Here's how the part is built. I have some questions about the finished solid (model axes, mm). Face numbers are marked on the shaded views. Coordinates: 2 decimals unless noted, no trailing zeros. Write each loop counter-clockwise with the first axis right and the second up, starting at its lowest first coordinate (ties: lowest second). Pieces come first, ordered by that corner, then holes. Notation, with made-up numbers: (7, 66) -> (66, 66) arc R12 ccw to (66, 86) -> close; hole circle Ø7 at (-7, 36.5). An arc over 180 degrees is marked (long way). Put each result on its own line as item: value. Start each with the question number.
Item 1: I want a section at D-D, the plane x = 113. List the corners of the cut face in (y, z) for me, then the cut area to 3 significant figures.
Item 2: If we mould it in two halves opening along Y, with no side actions, what happens to the marked faces 1 and 2? For each: released by +Y, released by -Y, zero draft, split by the parting line, or undercut.
Item 3: I want a section at C-C, the plane y = 32. List the corners of the cut face in (x, z) for me.
Item 4: For pin 1 (2 mm diameter, centred on x = 151.5, y = 38.5, fed in from -Z); pin 2 (10 mm diameter, centred on x = 61, y = 61.5, fed in from -Z), each with a flat end and sliding along its axis, tell me the tip position at first contact or that it passes through.
Item 5: I want a section at A-A, the plane x = 18. List the corners of the cut face in (y, z) for me, then the cut area to 3 significant figures.
Item 6: I want a section at B-B, the plane z = 3. State how many separate pieces and enclosed holes the cut face has, then the cut area to 3 significant figures.
Item 7: I need wall thicknesses on line 1 (Y direction, x = 27.75, z = 2.25); line 2 (X direction, y = 63, z = 4.75); line 3 (X direction, y = 16, z = 7.25). Which ranges of each line are inside material? Lowest first, please. Write a range as [from, to].
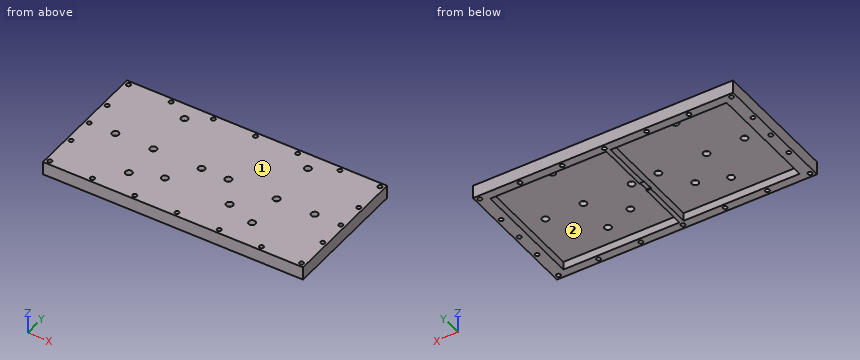
from build123d import *

# Parameters (mm, degrees)
F0_W      = 154
F0_H      = 77
F1_DEPTH  = 7.873
F2_W      = 140
F2_H      = 67
F3_DEPTH  = 4.873
F4_R      = 1.25
F5_DEPTH  = 7.873
F6_R      = 1.25
F7_DEPTH  = 7.873
F8_R      = 1.25
F9_DEPTH  = 7.873
F10_R     = 1.25
F11_DEPTH = 7.873
F12_R     = 1.25
F13_DEPTH = 7.873
F14_R     = 1.25
F15_DEPTH = 7.873
F16_R     = 1.25
F17_DEPTH = 7.873
F18_R     = 1.25
F19_DEPTH = 7.873
F20_R     = 1.25
F21_DEPTH = 7.873
F22_R     = 1.25
F23_DEPTH = 7.873
F24_R     = 1.25
F25_DEPTH = 7.873
F26_R     = 1.25
F27_DEPTH = 7.873
F28_R     = 1.25
F29_DEPTH = 7.873
F30_R     = 1.25
F31_DEPTH = 7.873
F32_R     = 1.25
F33_DEPTH = 7.873
F34_R     = 1.25
F35_DEPTH = 7.873
F36_R     = 1.25
F37_DEPTH = 7.873
F38_R     = 1.25
F39_DEPTH = 7.873
F40_R     = 1.25
F41_DEPTH = 7.873
F42_R     = 1.25
F43_DEPTH = 7.873
F44_R     = 2
F45_DEPTH = 3
F46_R     = 2
F47_DEPTH = 3
F48_R     = 2
F49_DEPTH = 3
F50_R     = 2
F51_DEPTH = 3
F52_R     = 2
F53_DEPTH = 3
F54_R     = 2
F55_DEPTH = 3
F56_R     = 2
F57_DEPTH = 3
F58_R     = 2
F59_DEPTH = 3
F61_R     = 2
F62_DEPTH = 3
F64_R     = 2
F65_DEPTH = 3
F66_R     = 2
F67_DEPTH = 3
F63_R     = 2
F68_DEPTH = 3
F69_W     = 2.5
F69_H     = 67
F70_DEPTH = 4.873
F60_W     = 2.5
F60_H     = 6.7
F71_DEPTH = 0.723


with BuildPart() as f1:
    # F0 (on Top) → F1 (new body)
    with BuildSketch(Plane.XY):
        with Locations((77, 38.5)):
            Rectangle(F0_W, F0_H)
    extrude(amount=F1_DEPTH)

    # F2 (on Top) → F3 (cut)
    with BuildSketch(Plane.XY):
        with Locations((77, 38.5)):
            Rectangle(F2_W, F2_H)
    extrude(amount=F3_DEPTH, mode=Mode.SUBTRACT)

    # F4 (on face) → F5 (cut)
    with BuildSketch(Plane.XY.offset(7.873)):
        with Locations((2.5, 2.5)):
            Circle(F4_R)
    extrude(amount=-F5_DEPTH, mode=Mode.SUBTRACT)

    # F6 (on face) → F7 (cut)
    with BuildSketch(Plane.XY.offset(7.873)):
        with Locations((27.75, 2.5)):
            Circle(F6_R)
    extrude(amount=-F7_DEPTH, mode=Mode.SUBTRACT)

    # F8 (on face) → F9 (cut)
    with BuildSketch(Plane.XY.offset(7.873)):
        with Locations((52.75, 2.5)):
            Circle(F8_R)
    extrude(amount=-F9_DEPTH, mode=Mode.SUBTRACT)

    # F10 (on face) → F11 (cut)
    with BuildSketch(Plane.XY.offset(7.873)):
        with Locations((77.75, 2.5)):
            Circle(F10_R)
    extrude(amount=-F11_DEPTH, mode=Mode.SUBTRACT)

    # F12 (on face) → F13 (cut)
    with BuildSketch(Plane.XY.offset(7.873)):
        with Locations((102.75, 2.5)):
            Circle(F12_R)
    extrude(amount=-F13_DEPTH, mode=Mode.SUBTRACT)

    # F14 (on face) → F15 (cut)
    with BuildSketch(Plane.XY.offset(7.873)):
        with Locations((127.75, 2.5)):
            Circle(F14_R)
    extrude(amount=-F15_DEPTH, mode=Mode.SUBTRACT)

    # F16 (on face) → F17 (cut)
    with BuildSketch(Plane.XY.offset(7.873)):
        with Locations((151.5, 2.5)):
            Circle(F16_R)
    extrude(amount=-F17_DEPTH, mode=Mode.SUBTRACT)

    # F18 (on face) → F19 (cut)
    with BuildSketch(Plane.XY.offset(7.873)):
        with Locations((2.5, 22)):
            Circle(F18_R)
    extrude(amount=-F19_DEPTH, mode=Mode.SUBTRACT)

    # F20 (on face) → F21 (cut)
    with BuildSketch(Plane.XY.offset(7.873)):
        with Locations((151.5, 22)):
            Circle(F20_R)
    extrude(amount=-F21_DEPTH, mode=Mode.SUBTRACT)

    # F22 (on face) → F23 (cut)
    with BuildSketch(Plane.XY.offset(7.873)):
        with Locations((151.5, 38.5)):
            Circle(F22_R)
    extrude(amount=-F23_DEPTH, mode=Mode.SUBTRACT)

    # F24 (on face) → F25 (cut)
    with BuildSketch(Plane.XY.offset(7.873)):
        with Locations((2.5, 38.5)):
            Circle(F24_R)
    extrude(amount=-F25_DEPTH, mode=Mode.SUBTRACT)

    # F26 (on face) → F27 (cut)
    with BuildSketch(Plane.XY.offset(7.873)):
        with Locations((2.5, 55)):
            Circle(F26_R)
    extrude(amount=-F27_DEPTH, mode=Mode.SUBTRACT)

    # F28 (on face) → F29 (cut)
    with BuildSketch(Plane.XY.offset(7.873)):
        with Locations((151.5, 55)):
            Circle(F28_R)
    extrude(amount=-F29_DEPTH, mode=Mode.SUBTRACT)

    # F30 (on face) → F31 (cut)
    with BuildSketch(Plane.XY.offset(7.873)):
        with Locations((2.5, 74.5)):
            Circle(F30_R)
    extrude(amount=-F31_DEPTH, mode=Mode.SUBTRACT)

    # F32 (on face) → F33 (cut)
    with BuildSketch(Plane.XY.offset(7.873)):
        with Locations((151.5, 74.5)):
            Circle(F32_R)
    extrude(amount=-F33_DEPTH, mode=Mode.SUBTRACT)

    # F34 (on face) → F35 (cut)
    with BuildSketch(Plane.XY.offset(7.873)):
        with Locations((27.75, 74.5)):
            Circle(F34_R)
    extrude(amount=-F35_DEPTH, mode=Mode.SUBTRACT)

    # F36 (on face) → F37 (cut)
    with BuildSketch(Plane.XY.offset(7.873)):
        with Locations((127.75, 74.5)):
            Circle(F36_R)
    extrude(amount=-F37_DEPTH, mode=Mode.SUBTRACT)

    # F38 (on face) → F39 (cut)
    with BuildSketch(Plane.XY.offset(7.873)):
        with Locations((102.75, 74.5)):
            Circle(F38_R)
    extrude(amount=-F39_DEPTH, mode=Mode.SUBTRACT)

    # F40 (on face) → F41 (cut)
    with BuildSketch(Plane.XY.offset(7.873)):
        with Locations((52.75, 74.5)):
            Circle(F40_R)
    extrude(amount=-F41_DEPTH, mode=Mode.SUBTRACT)

    # F42 (on face) → F43 (cut)
    with BuildSketch(Plane.XY.offset(7.873)):
        with Locations((77.75, 74.5)):
            Circle(F42_R)
    extrude(amount=-F43_DEPTH, mode=Mode.SUBTRACT)

    # F44 (on face) → F45 (cut)
    with BuildSketch(Plane.XY.offset(7.873)):
        with Locations((40.5, 67.1)):
            Circle(F44_R)
    extrude(amount=-F45_DEPTH, mode=Mode.SUBTRACT)

    # F46 (on face) → F47 (cut)
    with BuildSketch(Plane.XY.offset(7.873)):
        with Locations((18, 38.5)):
            Circle(F46_R)
    extrude(amount=-F47_DEPTH, mode=Mode.SUBTRACT)

    # F48 (on face) → F49 (cut)
    with BuildSketch(Plane.XY.offset(7.873)):
        with Locations((69.1, 38.5)):
            Circle(F48_R)
    extrude(amount=-F49_DEPTH, mode=Mode.SUBTRACT)

    # F50 (on face) → F51 (cut)
    with BuildSketch(Plane.XY.offset(7.873)):
        with Locations((113.5, 67.1)):
            Circle(F50_R)
    extrude(amount=-F51_DEPTH, mode=Mode.SUBTRACT)

    # F52 (on face) → F53 (cut)
    with BuildSketch(Plane.XY.offset(7.873)):
        with Locations((84.9, 38.5)):
            Circle(F52_R)
    extrude(amount=-F53_DEPTH, mode=Mode.SUBTRACT)

    # F54 (on face) → F55 (cut)
    with BuildSketch(Plane.XY.offset(7.873)):
        with Locations((136, 38.5)):
            Circle(F54_R)
    extrude(amount=-F55_DEPTH, mode=Mode.SUBTRACT)

    # F56 (on face) → F57 (cut)
    with BuildSketch(Plane.XY.offset(7.873)):
        with Locations((57.8, 22.17)):
            Circle(F56_R)
    extrude(amount=-F57_DEPTH, mode=Mode.SUBTRACT)

    # F58 (on face) → F59 (cut)
    with BuildSketch(Plane.XY.offset(7.873)):
        with Locations((96.2, 22.17)):
            Circle(F58_R)
    extrude(amount=-F59_DEPTH, mode=Mode.SUBTRACT)

    # F61 (on face) → F62 (cut)
    with BuildSketch(Plane(origin=(0, 0, 4.873), x_dir=(1, 0, 0), z_dir=(0, 0, -1))):
        with Locations((40.5, -16)):
            Circle(F61_R)
    extrude(amount=-F62_DEPTH, mode=Mode.SUBTRACT)

    # F64 (on face) → F65 (cut)
    with BuildSketch(Plane(origin=(0, 0, 4.873), x_dir=(1, 0, 0), z_dir=(0, 0, -1))):
        with Locations((113.5, -38.5)):
            Circle(F64_R)
    extrude(amount=-F65_DEPTH, mode=Mode.SUBTRACT)

    # F66 (on face) → F67 (cut)
    with BuildSketch(Plane(origin=(0, 0, 4.873), x_dir=(1, 0, 0), z_dir=(0, 0, -1))):
        with Locations((113.5, -16)):
            Circle(F66_R)
    extrude(amount=-F67_DEPTH, mode=Mode.SUBTRACT)

    # F63 (on face) → F68 (cut)
    with BuildSketch(Plane(origin=(0, 0, 4.873), x_dir=(1, 0, 0), z_dir=(0, 0, -1))):
        with Locations((40.5, -38.5)):
            Circle(F63_R)
    extrude(amount=-F68_DEPTH, mode=Mode.SUBTRACT)

    # F69 (on face) → F70 (join)
    with BuildSketch(Plane(origin=(0, 0, 0), x_dir=(1, 0, 0), z_dir=(0, 0, -1))):
        with Locations((77, -38.5)):
            Rectangle(F69_W, F69_H)
    extrude(amount=-F70_DEPTH)

    # F60 (on face) → F71 (cut)
    with BuildSketch(Plane(origin=(0, 0, 0), x_dir=(1, 0, 0), z_dir=(0, 0, -1))):
        with Locations((77, -38.5)):
            Rectangle(F60_W, F60_H)
    extrude(amount=-F71_DEPTH, mode=Mode.SUBTRACT)


solid = f1.part
Calculated:
1. outline: (0, 0) -> (5, 0) -> (5, 4.87) -> (14.06, 4.87) -> (14.06, 7.87) -> (0, 7.87) -> close; (17.94, 4.87) -> (36.56, 4.87) -> (36.56, 7.87) -> (17.94, 7.87) -> close; (40.44, 4.87) -> (65.16, 4.87) -> (65.16, 7.87) -> (40.44, 7.87) -> close; (69.04, 4.87) -> (72, 4.87) -> (72, 0) -> (77, 0) -> (77, 7.87) -> (69.04, 7.87) -> close
1. area: 245 mm2
2. face 1: zero draft
2. face 2: undercut
3. outline: (0, 0) -> (7, 0) -> (7, 4.87) -> (75.75, 4.87) -> (75.75, 0) -> (78.25, 0) -> (78.25, 4.87) -> (147, 4.87) -> (147, 0) -> (154, 0) -> (154, 7.87) -> (0, 7.87) -> close
4. pin 1: passes through
4. pin 2: stops at z = 4.87
5. outline: (0, 0) -> (5, 0) -> (5, 4.87) -> (36.5, 4.87) -> (36.5, 7.87) -> (0, 7.87) -> close; (40.5, 4.87) -> (72, 4.87) -> (72, 0) -> (77, 0) -> (77, 7.87) -> (40.5, 7.87) -> close
5. area: 268 mm2
6. separate pieces: 1
6. enclosed holes: 22
6. area: 2,550 mm2
7. line 1: y = [0, 1.25], [3.75, 5], [72, 73.25], [75.75, 77]
7. line 2: x = [0, 7], [75.75, 78.25], [147, 154]
7. line 3: x = [0, 38.5], [42.5, 111.5], [115.5, 154]
